from build123d import *

# Parameters (mm, degrees)
SKETCH1_W               = 43.18
SKETCH1_H               = 68.58
BOSS_EXTRUDE1_DEPTH     = 6.35
F_1_4_CLEARANCE_HOLE1_D = 6.7564
SKETCH7_R               = 2.5
CUT_EXTRUDE1_DEPTH      = 7.35
CHAMFER1_SIZE           = 0.127


with BuildPart() as part:
    # Sketch1 → Boss-Extrude1 (new body)
    with BuildSketch(Plane(origin=(0, 0, 0), x_dir=(1, 0, 0), z_dir=(0, 1, 0))):
        Rectangle(SKETCH1_W, SKETCH1_H)
    extrude(amount=BOSS_EXTRUDE1_DEPTH)

    # 1/4 Clearance Hole1 (through all)
    with Locations(Plane(origin=(0, 6.35, 0), x_dir=(1, 0, 0), z_dir=(0, 1, 0))):
        with Locations((15.24, -21.59), (-15.24, -21.59)):
            Hole(F_1_4_CLEARANCE_HOLE1_D / 2)

    # Sketch7 → Cut-Extrude1 (cut, through all)
    with BuildSketch(Plane.XZ):
        with Locations((0, -12.31)):
            Circle(SKETCH7_R)
    extrude(amount=-CUT_EXTRUDE1_DEPTH, mode=Mode.SUBTRACT)

    # Chamfer1
    chamfer1_edges = [part.edges().sort_by_distance(p)[0] for p in [
        (-2.5, 6.35, -12.31),
        (-2.5, 0, -12.31),
    ]]
    chamfer(chamfer1_edges, length=CHAMFER1_SIZE)


solid = part.part
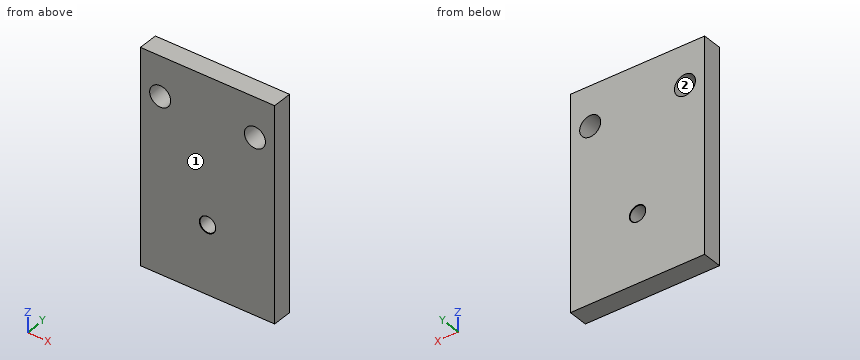
Build history of the part. All positions in model axes, mm. Face numbers are marked on the shaded views. Round coordinates to 2 decimals unless told otherwise and drop trailing zeros. Write each loop counter-clockwise with the first axis right and the second up, starting at its lowest first coordinate (ties: lowest second). Pieces come first, ordered by that corner, then holes. Notation, with made-up numbers: (82, -39) - (110, -39) arc R13 ccw to (110, -26) - close; hole circle Ø9 at (5, -1). An arc over 180 degrees is marked (long way). One line per question, with ' | ' between items.
1. Band-saw the part on C-C, the plane y = 4. Write the cut outline in (x, z).
Results are:
outline: (-21.59, -34.29) - (21.59, -34.29) - (21.59, 34.29) - (-21.59, 34.29) - close; hole circle Ø6.76 at (-15.24, 21.59); hole circle Ø5 at (0, -12.31); hole circle Ø6.76 at (15.24, 21.59)
2. Drop a flat-ended pin along its axis: pin 1 Ø4 at (x, z) = (-2, -2) entering from -Y. Give the stop position or say it passes through.
Results are:
pin 1: y = 0
3. Drill centre lines: line 1 along X through (y, z) = (4, 21.59); line 2 along Z through (x, y) = (0, 5); line 3 along Z through (x, y) = (15.24, 1.5). Where is each one in solid material? Low to high. Write a range as from..to.
Results are:
line 1: -21.59..-18.62, -11.86..11.86, 18.62..21.59 | line 2: -34.29..-14.81, -9.81..34.29 | line 3: -34.29..18.21, 24.97..34.29
4. Mould opens along X. For the marked faces 1 and 2 say: released by +X, released by -X, zero draft, split by the parting line, or undercut.
Results are:
face 1: zero draft | face 2: undercut
5. Band-saw the part on A-A, the plane x = 15.24. Write the cut outline in (y, z).
Results are:
outline: (0, -34.29) - (6.35, -34.29) - (6.35, 18.21) - (0, 18.21) - close; (0, 24.97) - (6.35, 24.97) - (6.35, 34.29) - (0, 34.29) - close
6. Band-saw the part on B-B, the plane z = -12.31. Write the cut outline in (x, y), and give its area (3 significant figures).
Results are:
outline: (-21.59, 0) - (-2.63, 0) - (-2.5, 0.13) - (-2.5, 6.22) - (-2.63, 6.35) - (-21.59, 6.35) - close; (2.5, 0.13) - (2.63, 0) - (21.59, 0) - (21.59, 6.35) - (2.63, 6.35) - (2.5, 6.22) - close | area: 242 mm^2
7. Band-saw the part on D-D, the plane z = 19.5. Write the cut outline in (x, y).
Results are:
outline: (-21.59, 0) - (-17.89, 0) - (-17.89, 6.35) - (-21.59, 6.35) - close; (-12.59, 0) - (12.59, 0) - (12.59, 6.35) - (-12.59, 6.35) - close; (17.89, 0) - (21.59, 0) - (21.59, 6.35) - (17.89, 6.35) - close
